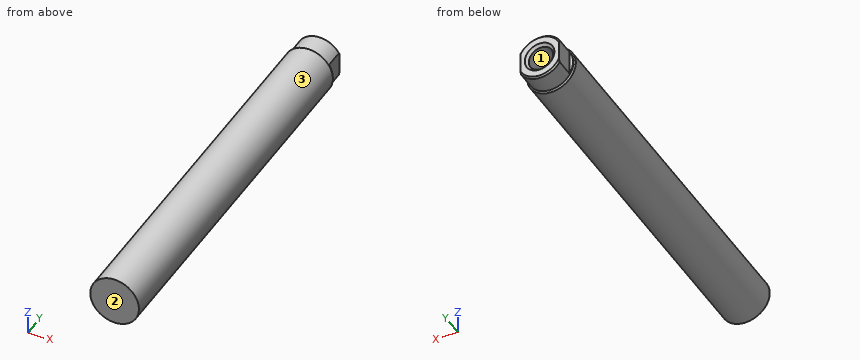
Autodesk Inventor part; units mm, degrees
ref_plane "b11_XY" through (0, 0, 0) normal (0, 1, 0) x (1, 0, 0)
ref_plane "b11_YZ" through (0, 0, 0) normal (1, 0, 0) x (0, 0, -1)
ref_plane "b11_ZX" through (0, 0, 0) normal (0, 0, -1) x (0, 1, 0)
sketch "Sketch_31" plane through (0, 0, 0) normal (0, 0, 1) x (1, 0, 0)
  line L0 (0, 0) -> (0, 63.7794)
  line L1 (0, 63.7794) -> (3.473, 63.7794)
  line L2 (3.473, 63.7794) -> (3.7211, 63.5313)
  line L3 (3.7211, 63.5313) -> (3.7211, 60.3504)
  line L4 (3.7211, 60.3504) -> (3.9688, 60.1028)
  line L5 (3.9688, 60.1028) -> (3.9688, 0)
  line L6 (3.9688, 0) -> (0, 0)
  line L7 (0, 0) -> (0, 63.7794)
revolve "Revolution1" add sketch "Sketch_31" angle 360 about axis through (0, 0, 0) along (0, -1, 0)
sketch "Sketch2" plane through (0, 63.7794, 0) normal (0, 1, 0) x (1, 0, 0)
  point P0 (0, 0)
hole "Hole1" at (0, 63.7794, 0) direction (0, -1, 0) diameter 3.9624 depth 12.9263 tip angle 120 countersink diameter 4.826 countersink angle 90
sketch "Sketch_29" plane through (0, 63.7794, 0) normal (0, 1, 0) x (1, 0, 0)
  line L0 (-6.2865, -15.875) -> (6.2865, -15.875)
  line L1 (6.2865, -15.875) -> (6.2865, 15.875)
  line L2 (6.2865, 15.875) -> (-6.2865, 15.875)
  line L3 (-6.2865, 15.875) -> (-6.2865, -15.875)
  line L4 (-3.1433, -7.9375) -> (3.1433, -7.9375)
  line L5 (3.1433, -7.9375) -> (3.1433, 7.9375)
  line L6 (3.1433, 7.9375) -> (-3.1433, 7.9375)
  line L7 (-3.1433, 7.9375) -> (-3.1433, -7.9375)
extrude "Extrusion1" cut sketch "Sketch_29" against normal blind 3.302
ref_plane "b11_XY" through (0, 0, 0) normal (0, 1, 0) x (1, 0, 0)
ref_plane "b11_YZ" through (0, 0, 0) normal (1, 0, 0) x (0, 0, -1)
ref_plane "b11_ZX" through (0, 0, 0) normal (0, 0, -1) x (0, 1, 0)
ref_plane "b2_XY" through (0, 63.7794, 0) normal (0, 1, 0) x (1, 0, 0)
ref_plane "b2_YZ" through (0, 63.7794, 0) normal (1, 0, 0) x (0, 0, -1)
ref_plane "b2_ZX" through (0, 63.7794, 0) normal (0, 0, -1) x (0, 1, 0)
ref_plane "f1_XY" through (0, 63.7794, 3.9688) normal (1, 0, 0) x (0, 0, -1)
ref_plane "f1_YZ" through (0, 63.7794, 3.9688) normal (0, 0, -1) x (0, 1, 0)
ref_plane "f1_ZX" through (0, 63.7794, 3.9688) normal (0, 1, 0) x (1, 0, 0)
ref_plane "f2_XY" through (0, 63.7794, -3.9688) normal (1, 0, 0) x (0, 0, -1)
ref_plane "f2_YZ" through (0, 63.7794, -3.9688) normal (0, 0, -1) x (0, 1, 0)
ref_plane "f2_ZX" through (0, 63.7794, -3.9688) normal (0, 1, 0) x (1, 0, 0)
ref_plane "h1_XY" through (-3.1433, 63.7794, 0) normal (0, 1, 0) x (1, 0, 0)
ref_plane "h1_YZ" through (-3.1433, 63.7794, 0) normal (1, 0, 0) x (0, 0, -1)
ref_plane "h1_ZX" through (-3.1433, 63.7794, 0) normal (0, 0, -1) x (0, 1, 0)
ref_plane "h2_XY" through (3.1433, 63.7794, 0) normal (0, 1, 0) x (1, 0, 0)
ref_plane "h2_YZ" through (3.1433, 63.7794, 0) normal (1, 0, 0) x (0, 0, -1)
ref_plane "h2_ZX" through (3.1433, 63.7794, 0) normal (0, 0, -1) x (0, 1, 0)
ref_plane "npt1_XY" through (0, 63.7794, 0) normal (0, 1, 0) x (1, 0, 0)
ref_plane "npt1_YZ" through (0, 63.7794, 0) normal (1, 0, 0) x (0, 0, -1)
ref_plane "npt1_ZX" through (0, 63.7794, 0) normal (0, 0, -1) x (0, 1, 0)
ref_plane "npt2_XY" through (0, 63.7794, 0) normal (0, 1, 0) x (1, 0, 0)
ref_plane "npt2_YZ" through (0, 63.7794, 0) normal (1, 0, 0) x (0, 0, -1)
ref_plane "npt2_ZX" through (0, 63.7794, 0) normal (0, 0, -1) x (0, 1, 0)
ref_plane "rod_XY" through (0, 63.7794, 0) normal (0, 1, 0) x (1, 0, 0)
ref_plane "rod_YZ" through (0, 63.7794, 0) normal (1, 0, 0) x (0, 0, -1)
ref_plane "rod_ZX" through (0, 63.7794, 0) normal (0, 0, -1) x (0, 1, 0)
ref_plane "rod_to_part_XY" through (0, 0, 0) normal (0, 1, 0) x (1, 0, 0)
ref_plane "rod_to_part_YZ" through (0, 0, 0) normal (1, 0, 0) x (0, 0, -1)
ref_plane "rod_to_part_ZX" through (0, 0, 0) normal (0, 0, -1) x (0, 1, 0)
ref_plane "th1_XY" through (0, 63.7794, 2.413) normal (0, 1, 0) x (1, 0, 0)
ref_plane "th1_YZ" through (0, 63.7794, 2.413) normal (1, 0, 0) x (0, 0, -1)
ref_plane "th1_ZX" through (0, 63.7794, 2.413) normal (0, 0, -1) x (0, 1, 0)
ref_plane "th2_XY" through (0, 63.7794, -2.413) normal (0, 1, 0) x (1, 0, 0)
ref_plane "th2_YZ" through (0, 63.7794, -2.413) normal (1, 0, 0) x (0, 0, -1)
ref_plane "th2_ZX" through (0, 63.7794, -2.413) normal (0, 0, -1) x (0, 1, 0)
ref_plane "to_rod_pivot_XY" through (0, 63.7794, 0) normal (0, 1, 0) x (1, 0, 0)
ref_plane "to_rod_pivot_YZ" through (0, 63.7794, 0) normal (1, 0, 0) x (0, 0, -1)
ref_plane "to_rod_pivot_ZX" through (0, 63.7794, 0) normal (0, 0, -1) x (0, 1, 0)
ref_plane "to_rod_pivot1_XY" through (0, 0, 0) normal (0, 1, 0) x (1, 0, 0)
ref_plane "to_rod_pivot1_YZ" through (0, 0, 0) normal (1, 0, 0) x (0, 0, -1)
ref_plane "to_rod_pivot1_ZX" through (0, 0, 0) normal (0, 0, -1) x (0, 1, 0)
properties part number "FO-042.5112.511-00_rod"
Verification items for the finished model (mm, model axes). Face numbers are marked on the shaded views. Coordinates: 2 decimals unless noted, no trailing zeros. Write each loop counter-clockwise with the first axis right and the second up, starting at its lowest first coordinate (ties: lowest second). Pieces come first, ordered by that corner, then holes. Notation, with made-up numbers: M 74,74 L 118,74 A7 cw 118,84 Z; hole C 44.25,39 d5. An arc over 180 degrees is marked long. Use a Markdown table: item, result.
Q1. Sectioned sample at A-A, the plane y = 9. Record the boundary of the cut face in (x, z).
Reply:
| item | result |
|---|---|
| outline | C 0,0 d7.94 |
Q2. Draft check along X on the marked faces 1, 2 and 3. Enter one of: +X half, -X half, draft (parallel to the pull), parting line (faces both ways), or undercut.
Reply:
| item | result |
|---|---|
| face 1 | undercut |
| face 2 | draft |
| face 3 | parting line |
Q3. Thickness scan on line 1 (Z direction, x = 0, y = 56.25); line 2 (Z direction, x = 0, y = 60.5); line 3 (Z direction, x = -1.5, y = 42). Record the ranges inside material, lowest first.
Reply:
| item | result |
|---|---|
| line 1 | z = -3.97 to -1.98, 1.98 to 3.97 |
| line 2 | z = -3.72 to -1.98, 1.98 to 3.72 |
| line 3 | z = -3.67 to 3.67 |
Q4. Go/stop test with flat-tipped pins: P1, Ø2.5, axis at x = 0, z = 0, coming from the +Y side; P2, Ø3, axis at x = 2.5, y = 9.5, coming from the +Z side; P3, Ø1.7, axis at y = 62.5, z = 1, coming from the +X side. Record where each tip stops, or that it passes through.
Reply:
| item | result |
|---|---|
| P1 | stops at y = 50.43 |
| P2 | stops at z = 3.84 |
| P3 | stops at x = 3.14 |
